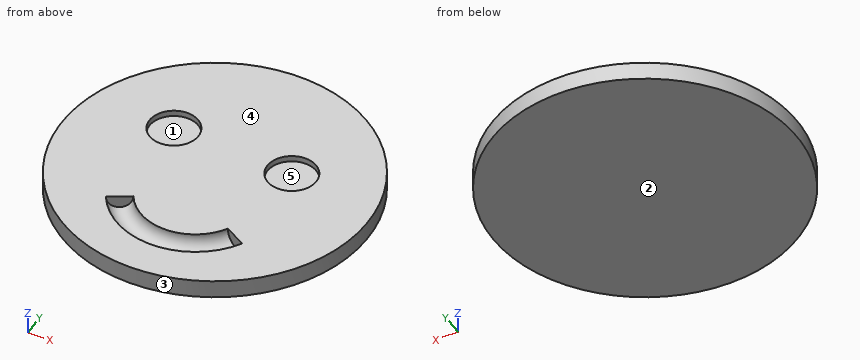
from build123d import *

# Parameters (mm, degrees)
TORUS_R               = 2
TORUS_ANGLE           = 120
TORUS_PLACEMENT_ANGLE = 150
CYLINDER002_R         = 4
CYLINDER002_DEPTH     = 4
CYLINDER001_R         = 4
CYLINDER001_DEPTH     = 4
CYLINDER_R            = 25
CYLINDER_DEPTH        = 3


with BuildPart() as torus:
    # Torus → Torus (revolve)
    with BuildSketch(Plane.XZ):
        with Locations((11, 0)):
            Circle(TORUS_R)
    revolve(axis=Axis((0, 0, 0), (0, 0, 1)), revolution_arc=TORUS_ANGLE)


with BuildPart() as torus_1:
    # Torus placement: moved
    add(torus.part.moved(Location((0, -6, 5))).rotate(Axis((0, -6, 5), (0, 0, -1)), TORUS_PLACEMENT_ANGLE))


with BuildPart() as cilindre002:
    # Cylinder002 → Cylinder002 (new body)
    with BuildSketch(Plane(origin=(10, 5, 2), x_dir=(1, 0, 0), z_dir=(0, 0, 1))):
        Circle(CYLINDER002_R)
    extrude(amount=CYLINDER002_DEPTH)


with BuildPart() as cilindre001:
    # Cylinder001 → Cylinder001 (new body)
    with BuildSketch(Plane(origin=(-10, 6, 2), x_dir=(1, 0, 0), z_dir=(0, 0, 1))):
        Circle(CYLINDER001_R)
    extrude(amount=CYLINDER001_DEPTH)


with BuildPart() as cut002:
    # Cylinder → Cylinder (new body)
    with BuildSketch(Plane.XY):
        Circle(CYLINDER_R)
    extrude(amount=CYLINDER_DEPTH)

    # Cut: cut Cilindre001
    add(cilindre001.part, mode=Mode.SUBTRACT)

    # Cut001: cut Cilindre002
    add(cilindre002.part, mode=Mode.SUBTRACT)


with BuildPart() as cut002_1:
    # Cut001 placement: moved
    add(cut002.part.moved(Location((0, 0, 2))))

    # Cut002: cut Torus
    add(torus_1.part, mode=Mode.SUBTRACT)


solid = cut002_1.part
CAD build for the part. Positions are in the model's coordinates, mm. Face numbers are marked on the shaded views. A direction names the side the tool comes from. Give positions to 0.01 mm unless a question says otherwise; leave off trailing zeros. Write each loop counter-clockwise with the first axis right and the second up, starting at its lowest first coordinate (ties: lowest second). Pieces come first, ordered by that corner, then holes. Notation, with made-up numbers: (48, 57) -> (68, 57) arc R25 cw to (68, 69) -> close; hole circle Ø11 at (54.25, 26.5). An arc over 180 degrees is marked (long way). Return JSON: item names as keys, results as strings.
Item 1: Band-saw the part on A-A (y = 5). List the corners of the cut face in (x, z).
Answer below:
{"outline": "(-24.49, 2) -> (24.49, 2) -> (24.49, 5) -> (14, 5) -> (14, 4) -> (6, 4) -> (6, 5) -> (-6.13, 5) -> (-6.13, 4) -> (-13.87, 4) -> (-13.87, 5) -> (-24.49, 5) -> close"}
Item 2: Two-plate mould, pull along X, no slides. Class the marked faces 3, 4 and 5: +X half, -X half, draft (parallel to the pull), parting line (faces both ways), or undercut.
Answer below:
{"face 3": "parting line", "face 4": "draft", "face 5": "undercut"}
Item 3: Drop flat-ended pins along their axis: pin 1 (1.5 mm diameter, centred on y = -14.5, z = 3, fed in from -X); pin 2 (1.5 mm diameter, centred on x = -19.5, y = 17.5, fed in from -Z). Give the stop position or say it passes through.
Answer below:
{"pin 1": "stops at x = -20.88", "pin 2": "passes through"}
Item 4: Band-saw the part on C-C (x = 12.5). List the corners of the cut face in (y, z).
Answer below:
{"outline": "(-21.65, 2) -> (21.65, 2) -> (21.65, 5) -> (8.12, 5) -> (8.12, 4) -> (1.88, 4) -> (1.88, 5) -> (-21.65, 5) -> close"}
Item 5: Tool access for the marked faces 1 and 2: list every direction of +Z, -Z, +X, -X, +Y, -Y with a clear straight run to the whole face (end or side of a thin tool).
Answer below:
{"face 1": "+Z", "face 2": "-Z, +X, -X, +Y, -Y"}
Item 6: Drill centre lines: probe 1 along Y at (x, z) = (-10, 4.55); probe 2 along Y at (x, z) = (10, 4.6); probe 3 along X at (y, z) = (-14, 4.25). Where is each one in solid material? Low to high.
Answer below:
{"probe 1": "y = -22.91 to -14.23, -11.77 to 2, 10 to 22.91", "probe 2": "y = -22.91 to -14.24, -11.77 to 1, 9 to 22.91", "probe 3": "x = -20.71 to -10.06, -4.43 to 4.43, 10.06 to 20.71"}
Item 7: Band-saw the part on B-B (x = -20). List the corners of the cut face in (y, z).
Answer below:
{"outline": "(-15, 2) -> (15, 2) -> (15, 5) -> (-15, 5) -> close"}
Item 8: Band-saw the part on D-D (y = 21). List the corners of the cut face in (x, z).
Answer below:
{"outline": "(-13.56, 2) -> (13.56, 2) -> (13.56, 5) -> (-13.56, 5) -> close"}
